Verification items for the finished model (mm, model axes). Round coordinates to 2 decimals unless told otherwise and drop trailing zeros. Write each loop counter-clockwise with the first axis right and the second up, starting at its lowest first coordinate (ties: lowest second). Pieces come first, ordered by that corner, then holes. Notation, with made-up numbers: (-37, -15) -> (-26, -15) arc R24 ccw to (-26, 12) -> close; hole circle Ø8 at (38.25, 6.5). An arc over 180 degrees is marked (long way). Use CSV: the item, a comma, the result in double quotes.
```python
from build123d import *

# Parameters (mm, degrees)
SKETCH1_W           = 90
SKETCH1_H           = 20
BOSS_EXTRUDE1_DEPTH = 3
CUT_EXTRUDE1_DEPTH  = 4
SKETCH3_R           = 1
CUT_EXTRUDE2_DEPTH  = 4


with BuildPart() as part:
    # Sketch1 → Boss-Extrude1 (new body)
    with BuildSketch(Plane(origin=(0, 0, 0), x_dir=(1, 0, 0), z_dir=(0, 1, 0))):
        with Locations((45, 10)):
            Rectangle(SKETCH1_W, SKETCH1_H)
    extrude(amount=BOSS_EXTRUDE1_DEPTH)

    # Sketch2 → Cut-Extrude1 (cut, through all)
    with BuildSketch(Plane(origin=(0, 3, 0), x_dir=(1, 0, 0), z_dir=(0, 1, 0))):
        with BuildLine():
            Line((90, 20), (10, 20))
            ThreePointArc((10, 20), (11.020288655, 19.947814386), (12.029928432, 19.791802212))
            Line((12.029928432, 19.791802212), (88, 12))
            ThreePointArc((88, 12), (89.414213562, 11.414213562), (90, 10))
            Line((90, 10), (90, 20))
        make_face()
        with BuildLine():
            Line((90, 0), (90, 10))
            ThreePointArc((90, 10), (89.414213562, 8.585786438), (88, 8))
            Line((88, 8), (12.029928432, 0.208197788))
            ThreePointArc((12.029928432, 0.208197788), (11.020288655, 0.052185614), (10, 0))
            Line((10, 0), (90, 0))
        make_face()
        with BuildLine():
            ThreePointArc((10, 0), (2.928932188, 2.928932188), (0, 10))
            Line((0, 10), (0, 0))
            Line((0, 0), (10, 0))
        make_face()
        with BuildLine():
            ThreePointArc((0, 10), (2.928932188, 17.071067812), (10, 20))
            Line((10, 20), (0, 20))
            Line((0, 20), (0, 10))
        make_face()
    extrude(amount=-CUT_EXTRUDE1_DEPTH, mode=Mode.SUBTRACT)

    # Sketch3 → Cut-Extrude2 (cut, through all)
    with BuildSketch(Plane(origin=(0, 3, 0), x_dir=(1, 0, 0), z_dir=(0, 1, 0))):
        with Locations((10, 10)):
            Circle(SKETCH3_R)
        with Locations((88, 10)):
            Circle(SKETCH3_R)
    extrude(amount=-CUT_EXTRUDE2_DEPTH, mode=Mode.SUBTRACT)


solid = part.part
```
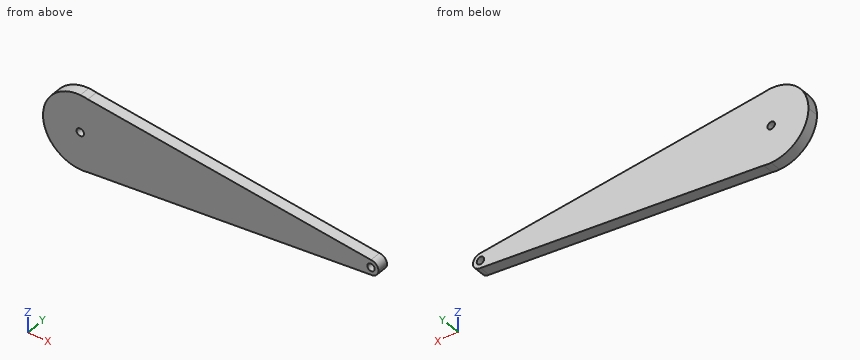
Q1. Section check C-C (x = 60). Record the cut outline in (y, z), plus the area to 3 significant figures.
Filled in:
outline,"(0, -14.87) -> (3, -14.87) -> (3, -5.13) -> (0, -5.13) -> close"
area,"29.2 mm²"
Q2. Section check A-A (y = 1). Record the cut outline in (x, z).
Filled in:
outline,"(12.03, -19.79) -> (88, -12) arc R2 ccw to (88, -8) -> (12.03, -0.21) arc R10 ccw (long way) to start; hole circle Ø2 at (10, -10); hole circle Ø2 at (88, -10)"
Q3. Section check B-B (z = -2). Record the cut outline in (x, y).
Filled in:
outline,"(4, 0) -> (29.5, 0) -> (29.5, 3) -> (4, 3) -> close"
Q4. Go/stop test with a flat-tipped pin: P1, Ø1.6, axis at x = 10, z = -10, coming from the -Y side. Record where the tip stops, or that it passes through.
Filled in:
P1,"through"
Q5. Material ranges on L1, parallel to X at y = 1.2, z = -10; L2, parallel to Z at x = 10, y = 1.2; L3, parallel to Z at x = 88, y = 1.35, recorded low to high.
Filled in:
L1,"0 to 9, 11 to 87, 89 to 90"
L2,"-20 to -11, -9 to 0"
L3,"-12 to -11, -9 to -8"
